Build history of the part. All positions in model axes, mm. A direction names the side the tool comes from. Round coordinates to 2 decimals unless told otherwise and drop trailing zeros. Write each loop counter-clockwise with the first axis right and the second up, starting at its lowest first coordinate (ties: lowest second). Pieces come first, ordered by that corner, then holes. Notation, with made-up numbers: (87, 33) - (132, 33) arc R14 cw to (132, 45) - close; hole circle Ø5 at (-37, -33). An arc over 180 degrees is marked (long way). Write each question's results on one line, items separated by ' | '.
from build123d import *

# Parameters (mm, degrees)
F1_DEPTH = 0.762
F2_DEPTH = 1.778


with BuildPart() as f1:
    # F0 (on Front) → F1 (new body)
    with BuildSketch(Plane.XZ):
        Polygon((-2.501412, 0.441066), (-3.909187, -7.542823), (8.829997, -7.542823), (9.712129, -2.54), (70.679427, -2.54), (79.377093, 47.603999), (56.517093, 47.603999), (55.642641, 42.562587), (17.664932, 42.562587), (18.553869, 47.603999), (5.814686, 47.603999), align=None)
        Polygon((-0.882133, -5.002823), (0, 0), (6.174929, 35.019764), (13.794929, 35.019764), (12.892384, 29.901175), (7.62, 0), (6.737867, -5.002823), align=None, mode=Mode.SUBTRACT)
        Polygon((10.16, 0), (15.432384, 29.901175), (25.592384, 29.901175), (26.03345, 32.402587), (15.87345, 32.402587), (17.217062, 40.022587), (34.997062, 40.022587), (27.94, 0), align=None, mode=Mode.SUBTRACT)
        Polygon((48.26, 0), (30.48, 0), (37.537062, 40.022587), (55.317062, 40.022587), (52.012466, 21.281294), (44.392466, 21.281294), (46.35345, 32.402587), (43.81345, 32.402587), (39.443612, 7.62), (41.983612, 7.62), (43.944596, 18.741294), (51.564596, 18.741294), align=None, mode=Mode.SUBTRACT)
        Polygon((14.2428, 37.559764), (6.6228, 37.559764), (7.945999, 45.063999), (15.565999, 45.063999), align=None, mode=Mode.SUBTRACT)
        Polygon((50.8, 0), (58.61652, 45.063999), (66.23652, 45.063999), (63.870264, 31.421999), (66.410264, 31.421999), (68.77652, 45.063999), (76.39652, 45.063999), (72.708546, 23.801999), (62.548546, 23.801999), (62.107974, 21.261999), (72.267974, 21.261999), (68.58, 0), (60.96, 0), (63.326256, 13.641999), (60.786256, 13.641999), (58.42, 0), align=None, mode=Mode.SUBTRACT)
        Polygon((24.058858, 21.204117), (21.518858, 21.204117), (19.313526, 8.697058), (21.853526, 8.697058), align=None)
    extrude(amount=F1_DEPTH)

    # F0 (on Front) → F2 (join)
    with BuildSketch(Plane.XZ):
        Polygon((6.174929, 35.019764), (0, 0), (7.62, 0), (12.892384, 29.901175), (13.794929, 35.019764), align=None)
        Polygon((7.62, 0), (0, 0), (-0.882133, -5.002823), (6.737867, -5.002823), align=None)
        Polygon((7.945999, 45.063999), (6.6228, 37.559764), (14.2428, 37.559764), (15.565999, 45.063999), align=None)
        Polygon((25.592384, 29.901175), (15.432384, 29.901175), (10.16, 0), (27.94, 0), (34.997062, 40.022587), (17.217062, 40.022587), (15.87345, 32.402587), (26.03345, 32.402587), align=None)
        Polygon((19.313526, 8.697058), (21.518858, 21.204117), (24.058858, 21.204117), (21.853526, 8.697058), align=None, mode=Mode.SUBTRACT)
        Polygon((37.537062, 40.022587), (30.48, 0), (48.26, 0), (51.564596, 18.741294), (43.944596, 18.741294), (41.983612, 7.62), (39.443612, 7.62), (43.81345, 32.402587), (46.35345, 32.402587), (44.392466, 21.281294), (52.012466, 21.281294), (55.317062, 40.022587), align=None)
        Polygon((66.23652, 45.063999), (58.61652, 45.063999), (50.8, 0), (58.42, 0), (60.786256, 13.641999), (63.326256, 13.641999), (60.96, 0), (68.58, 0), (72.267974, 21.261999), (62.107974, 21.261999), (62.548546, 23.801999), (72.708546, 23.801999), (76.39652, 45.063999), (68.77652, 45.063999), (66.410264, 31.421999), (63.870264, 31.421999), align=None)
    extrude(amount=F2_DEPTH)


solid = f1.part
(1) Tool access for faces 1 (the flat face through (61, -1.778, 23)), 2 (the flat face through (67.61, -1.26, 38.34)), 3 (the flat face through (70.4, -1.3, 10.5)), 4 (the flat face through (74.967, -0.376, 22.181)), 5 (the flat face through (22, -0.762, 15)): list every direction of +Z, -Z, +X, -X, +Y, -Y with a clear straight run to the whole face (end or side of a thin tool).
Worked answers:
face 1: +Z, -Z, +X, -X, -Y | face 2: +Z, -Y | face 3: -Z, +X, -Y | face 4: -Z, +X, +Y, -Y | face 5: -Y
(2) Flat gauge pins, fed straight in: pin 1 Ø5 at (x, z) = (41, 16.5) entering from +Y; pin 2 Ø0.8 at (x, y) = (47, -1.5) entering from -Z; pin 3 Ø0.5 at (x, y) = (47, -1.5) entering from +Z. Where does each tip first touch, or does it go through?
Worked answers:
pin 1: stops at y = 0 | pin 2: stops at z = 0 | pin 3: stops at z = 40.02
(3) Drill centre lines: probe 1 along X at (y, z) = (-1.1, 38); probe 2 along X at (y, z) = (-0.95, 5.5); probe 3 along X at (y, z) = (-1.6, 17). Where is each one in solid material? Low to high. Write a range as [from, to].
Worked answers:
probe 1: x = [6.7, 14.32], [16.86, 34.64], [37.18, 54.96], [57.39, 65.01], [67.55, 75.17] | probe 2: x = [0.97, 8.59], [11.13, 28.91], [31.45, 49.23], [51.75, 59.37], [61.91, 69.53] | probe 3: x = [3, 10.62], [13.16, 20.78], [23.32, 30.94], [33.48, 41.1], [43.64, 51.26], [53.75, 71.53]
(4) Slice it at B-B, the plane y = -1.45. State how many separate pieces and enclosed holes the cut face has, and give its area (3 significant figures).
Worked answers:
separate pieces: 5 | enclosed holes: 1 | area: 2,350 mm2
(5) Slice it at A-A, the plane z = 43.5. Write the cut outline in (x, y).
Worked answers:
outline: (5.09, -0.76) - (7.67, -0.76) - (7.67, -1.78) - (15.29, -1.78) - (15.29, -0.76) - (17.83, -0.76) - (17.83, 0) - (5.09, 0) - close; (55.81, -0.76) - (58.35, -0.76) - (58.35, -1.78) - (65.97, -1.78) - (65.97, -0.76) - (68.51, -0.76) - (68.51, -1.78) - (76.13, -1.78) - (76.13, -0.76) - (78.67, -0.76) - (78.67, 0) - (55.81, 0) - close
(6) Two-plate mould, pull along X, no slides. Class faces 6 (the flat face through (74.527, -1.263, 34.284)), 7 (the flat face through (20.4, -1.26, 14.86)), 8 (the flat face through (40, -1.778, 20)): released by +X, released by -X, zero draft, split by the parting line, or undercut.
Worked answers:
face 6: released by +X | face 7: undercut | face 8: zero draft
(7) Slice it at C-C, the plane x = 41. Write the cut outline in (y, z), and give its area (3 significant figures).
Worked answers:
outline: (-1.78, 0) - (-0.76, 0) - (-0.76, -2.54) - (0, -2.54) - (0, 42.56) - (-0.76, 42.56) - (-0.76, 40.02) - (-1.78, 40.02) - (-1.78, 16.45) - (-0.76, 16.45) - (-0.76, 7.62) - (-1.78, 7.62) - close | area: 66.1 mm2
